```python
from build123d import *

# Parameters (mm, degrees)
F0_W           = 304.8
F0_H           = 6.35
F1_DEPTH       = 38.1
F3_D           = 2.7051
F3_DEPTH       = 15.08125
F3_TIP         = 0.8126940303
F5_D           = 3.2639
F5_CSINK_D     = 6.477
F5_CSINK_ANGLE = 82
F7_DEPTH       = 25.4


with BuildPart() as f1:
    # F0 (on Top) → F1 (new body)
    with BuildSketch(Plane.XY):
        Rectangle(F0_W, F0_H)
    extrude(amount=F1_DEPTH)

    # F3
    with Locations(Plane(origin=(0, 0, 0), x_dir=(1, 0, 0), z_dir=(0, 0, -1))):
        with Locations((-127, 0), (127, 0), (25.4, 0)):
            Hole(F3_D / 2, depth=F3_DEPTH)
            with Locations((0, 0, -(F3_DEPTH + F3_TIP / 2))):  # 118° drill point
                Cone(0, F3_D / 2, F3_TIP, mode=Mode.SUBTRACT)

    # F5 (through all)
    with Locations(Plane(origin=(0, 3.175, 0), x_dir=(-1, 0, 0), z_dir=(0, 1, 0))):
        with Locations((-149.225, 25.4), (-149.225, 12.7), (149.225, 25.4), (149.225, 12.7)):
            CounterSinkHole(F5_D / 2, F5_CSINK_D / 2, counter_sink_angle=F5_CSINK_ANGLE)

    # F6 (on face) → F7 (cut)
    with BuildSketch(Plane(origin=(0, 3.175, 0), x_dir=(-1, 0, 0), z_dir=(0, 1, 0))):
        with BuildLine():
            Line((10.6065911112, 26.035), (-10.6065911112, 26.035))
            ThreePointArc((-10.6065911112, 26.035), (-12.7, 19.05), (-10.6065911112, 12.065))
            Line((-10.6065911112, 12.065), (10.6065911112, 12.065))
            ThreePointArc((10.6065911112, 12.065), (12.7, 19.05), (10.6065911112, 26.035))
        make_face()
        with BuildLine():
            Line((65.5934088888, 12.065), (86.8065911112, 12.065))
            ThreePointArc((86.8065911112, 12.065), (88.9, 19.05), (86.8065911112, 26.035))
            Line((86.8065911112, 26.035), (65.5934088888, 26.035))
            ThreePointArc((65.5934088888, 26.035), (63.5, 19.05), (65.5934088888, 12.065))
        make_face()
    extrude(amount=-F7_DEPTH, mode=Mode.SUBTRACT)


solid = f1.part
```
The model under review builds one solid part; all positions refer to its coordinate system, in mm. A direction names the side the tool comes from. Coordinates: 2 decimals unless noted, no trailing zeros. Order: outer loops, then holes, each group sorted by start corner. A loop starts at its lowest first (then second) coordinate and runs counter-clockwise, first axis right, second up. Notation, with made-up numbers: (77.5, -22) -> (86.5, -22) arc R18 ccw to (86.5, 1) -> close; hole circle Ø4 at (88, -38.75). An arc over 180 degrees is marked (long way). Answer in a Markdown table with one row per item. Add a question column.
Item 1: We need section A-A on x = -3. Write out the cut boundary in (y, z) (3 decimals).
Item 2: Machinability: for faces 4 (the cylindrical face through (-63.5, 0, 19.2)), 5 (the flat face through (152.4, 0, 19)), which of the approach directions +Z, -Z, +X, -X, +Y, -Y give a long, thin tool a straight path to every point of the face, cutting with its end or side? Answer none if there is none.
Item 3: Mouldability with a two-part tool opening along Z and no side actions: class faces 1 (the flat face through (-2, 3.175, 27)), 2 (the cylindrical face through (12.7, 0, 19.2)), 3 (the flat face through (-2, 0, 0)) as +Z half, -Z half, draft (parallel to the pull), parting line (faces both ways), or undercut.
Item 4: To check wall thickness, follow probe 1 along X at (y, z) = (0, 20); probe 2 along Z at (x, y) = (-84.5, -0.25) (3 decimals); probe 3 along X at (y, z) = (-0.5, 9). State the ranges of each line that lie inside material, in increasing order.
Item 5: Clearance check with flat-ended pins moving along their axes: pin 1 (2 mm diameter, centred on x = 127, y = 0, fed in from -Z); pin 2 (1.9 mm diameter, centred on x = -1, y = 1, fed in from -Z); pin 3 (2.5 mm diameter, centred on x = -149.225, z = 25.4, fed in from -Y). State where each tip first meets the part, or that it passes through.
Final values:
| question | item | result |
|---|---|---|
| 1 | outline | (-3.175, 0) -> (3.175, 0) -> (3.175, 12.065) -> (-3.175, 12.065) -> close; (-3.175, 26.035) -> (3.175, 26.035) -> (3.175, 38.1) -> (-3.175, 38.1) -> close |
| 2 | face 4 | +Y, -Y |
| 2 | face 5 | +Z, -Z, +X, +Y, -Y |
| 3 | face 1 | draft |
| 3 | face 2 | undercut |
| 3 | face 3 | -Z half |
| 4 | probe 1 | x = -152.4 to -88.86, -63.54 to -12.66, 12.66 to 152.4 |
| 4 | probe 2 | z = 0 to 12.065, 26.035 to 38.1 |
| 4 | probe 3 | x = -152.4 to -128.26, -125.74 to 24.14, 26.66 to 125.74, 128.26 to 152.4 |
| 5 | pin 1 | stops at z = 15.29 |
| 5 | pin 2 | stops at z = 0 |
| 5 | pin 3 | passes through |
